For this review, take the finished solid that the model builds, in its own axes (mm). A direction names the side the tool comes from. Round coordinates to 2 decimals unless told otherwise and drop trailing zeros. Write each loop counter-clockwise with the first axis right and the second up, starting at its lowest first coordinate (ties: lowest second). Pieces come first, ordered by that corner, then holes. Notation, with made-up numbers: M -40,79.5 L 18,79.5 A15 ccw 18,88.5 Z; hole C 43,35 d6. An arc over 180 degrees is marked long. One line per question, with ' | ' between items.
```python
from build123d import *

# Parameters (mm, degrees)
SKETCH1_W                  = 558.8
SKETCH1_H                  = 50.8
EXTRUDE1_DEPTH             = 12.7
CUT_EXTRUDE3_REACH         = 27.4
FILLET2_R                  = 9.525
M8X1_25_TAPPED_HOLE1_D     = 6.8
M8X1_25_TAPPED_HOLE1_DEPTH = 19.812
M8X1_25_TAPPED_HOLE1_TIP   = 2.042926105
M8X1_25_TAPPED_HOLE2_D     = 6.8
M8X1_25_TAPPED_HOLE2_DEPTH = 19.812
M8X1_25_TAPPED_HOLE2_TIP   = 2.042926105
CHAMFER1_SIZE              = 6.35


with BuildPart() as part:
    # Sketch1 → Extrude1 (new body, symmetric)
    with BuildSketch(Plane.XY):
        Rectangle(SKETCH1_W, SKETCH1_H)
    extrude(amount=EXTRUDE1_DEPTH, both=True)

    # Sketch4 → Cut-Extrude3 (cut, up to next)
    with BuildSketch(Plane.XY.offset(12.7), mode=Mode.PRIVATE) as cut_extrude3_sk1:
        with BuildLine():
            Line((-4.365625, -25.4), (-4.365625, 0))
            ThreePointArc((-4.365625, 0), (0, 4.365625), (4.365625, 0))
            Line((4.365625, 0), (4.365625, -25.4))
            ThreePointArc((4.365625, -25.4), (0, -29.765625), (-4.365625, -25.4))
        make_face()
    cut_extrude3_tool1 = extrude(cut_extrude3_sk1.sketch, amount=-CUT_EXTRUDE3_REACH, mode=Mode.PRIVATE) & part.part
    add(cut_extrude3_tool1.solids().sort_by_distance((0, -12.7, 12.7))[0], mode=Mode.SUBTRACT)

    # Fillet2
    fillet2_edges = [part.edges().sort_by_distance(p)[0] for p in [
        (-4.365625, -25.4, 0),
        (4.365625, -25.4, 0),
    ]]
    fillet(fillet2_edges, radius=FILLET2_R)

    # M8x1.25 Tapped Hole1
    with Locations(Plane(origin=(279.4, 0, 0), x_dir=(0, 0, -1), z_dir=(1, 0, 0))):
        with Locations((6.35, 12.7), (6.35, -12.7)):
            Hole(M8X1_25_TAPPED_HOLE1_D / 2, depth=M8X1_25_TAPPED_HOLE1_DEPTH)
            with Locations((0, 0, -(M8X1_25_TAPPED_HOLE1_DEPTH + M8X1_25_TAPPED_HOLE1_TIP / 2))):  # 118° drill point
                Cone(0, M8X1_25_TAPPED_HOLE1_D / 2, M8X1_25_TAPPED_HOLE1_TIP, mode=Mode.SUBTRACT)

    # M8x1.25 Tapped Hole2
    with Locations(Plane.ZY.offset(279.4)):
        with Locations((-6.35, 12.7), (-6.35, -12.7)):
            Hole(M8X1_25_TAPPED_HOLE2_D / 2, depth=M8X1_25_TAPPED_HOLE2_DEPTH)
            with Locations((0, 0, -(M8X1_25_TAPPED_HOLE2_DEPTH + M8X1_25_TAPPED_HOLE2_TIP / 2))):  # 118° drill point
                Cone(0, M8X1_25_TAPPED_HOLE2_D / 2, M8X1_25_TAPPED_HOLE2_TIP, mode=Mode.SUBTRACT)

    # Chamfer1
    chamfer1_edges = [part.edges().sort_by_distance(p)[0] for p in [
        (0, 25.4, 12.7),
    ]]
    chamfer(chamfer1_edges, length=CHAMFER1_SIZE)


solid = part.part
```
Item 1: Insertion check: pin 1 Ø3 at (x, z) = (62.5, 8) entering from +Y; pin 2 Ø5.5 at (y, z) = (12.7, -6.35) entering from -X. Each pin has a flat end and moves straight along its axis. Give the tip position at first contact, or say it passes through.
Results:
pin 1: y = 25.25 | pin 2: x = -259.2
Item 2: Machinability: for faces 1 (the face through (7.23, -22.684, -0.178)), 2 (the face through (-4, 25.4, -3)), which of the approach directions +Z, -Z, +X, -X, +Y, -Y give a long, thin tool a straight path to every point of the face, cutting with its end or side? Answer none if there is none.
Results:
face 1: +Z, -Z, -Y | face 2: +Z, -Z, +X, -X, +Y
Item 3: Mouldability with a two-part tool opening along X and no side actions: class faces 3 (the face through (-7.23, -22.684, -0.178)), 4 (the face through (-279.4, 0, 0)), 5 (the face through (145, -25.4, 0)) as +X half, -X half, draft (parallel to the pull), parting line (faces both ways), or undercut.
Results:
face 3: undercut | face 4: -X half | face 5: draft
Item 4: Take a section at A-A (x = -92.5). Write out the cut boundary in (y, z), then the cut area to 3 significant figures.
Results:
outline: M -25.4,-12.7 L 25.4,-12.7 L 25.4,6.35 L 19.05,12.7 L -25.4,12.7 Z | area: 1,270 mm2
Item 5: To check wall thickness, follow line 1 along Y through (x, z) = (268.25, -6.35); line 2 along Z through (x, y) = (271, -12.7); line 3 along X through (y, z) = (-13, -2). State the ranges of each line that lie inside material, in increasing order. Write a range as from..to.
Results:
line 1: -25.4..-16.1, -9.3..9.3, 16.1..25.4 | line 2: -12.7..-9.75, -2.95..12.7 | line 3: -279.4..-4.37, 4.37..279.4
